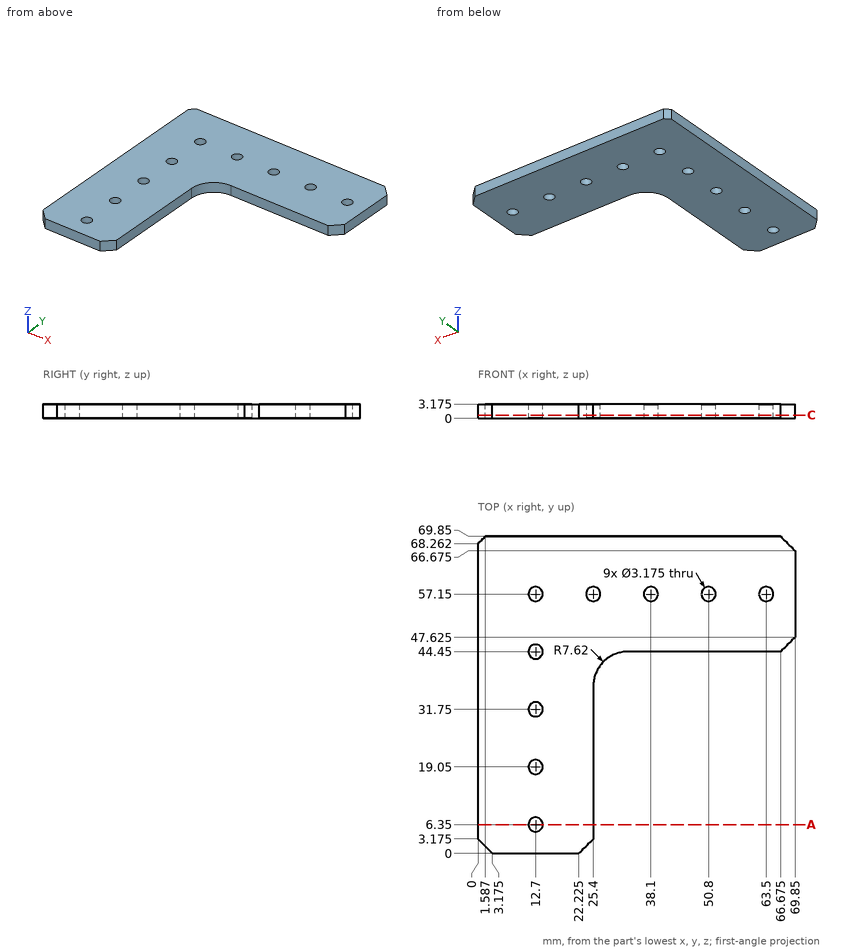
Job drawing, mm, ordinate dimensions from the low corner. One solid piece. Round coordinates to 2 decimals unless told otherwise and drop trailing zeros. Loops run counter-clockwise (first coordinate to the right, second up) from the corner with the lowest first, then second, coordinate; pieces in that order, holes last.
(1) Drop a flat-ended pin along its axis: pin 1 (1 mm diameter, centred on y = 15, z = 2.5, fed in from -X). Give the stop position or say it passes through.
(2) Cut at C-C (z = 0.7). State how many separate pieces and enclosed holes the cut face has, plus the area to 3 significant figures.
(3) Cut at A-A (y = 6.35). Give the cut face in (x, z) (1 decimal).
(4) Wall check: line 1 along Y through (x, z) = (12.7, 1.4); line 2 along X through (y, z) = (57.15, 1.35); line 3 along X through (y, z) = (57.5, 1.45). Give the ranges that are in metal, low to high.
Findings below:
1. pin 1: stops at x = 0
2. separate pieces: 1
2. enclosed holes: 9
2. area: 2,820 mm2
3. outline: (0, 0) - (11.1, 0) - (11.1, 3.2) - (0, 3.2) - close; (14.3, 0) - (25.4, 0) - (25.4, 3.2) - (14.3, 3.2) - close
4. line 1: y = 0 to 4.76, 7.94 to 17.46, 20.64 to 30.16, 33.34 to 42.86, 46.04 to 55.56, 58.74 to 69.85
4. line 2: x = 0 to 11.11, 14.29 to 23.81, 26.99 to 36.51, 39.69 to 49.21, 52.39 to 61.91, 65.09 to 69.85
4. line 3: x = 0 to 11.15, 14.25 to 23.85, 26.95 to 36.55, 39.65 to 49.25, 52.35 to 61.95, 65.05 to 69.85
